from build123d import *

# Parameters (mm, degrees)
SKETCH1_W           = 40
SKETCH1_H           = 70
BOSS_EXTRUDE2_DEPTH = 9
SKETCH3_W           = 20
SKETCH3_H           = 40
CUT_EXTRUDE1_DEPTH  = 42.303752856
SKETCH4_R           = 1.5
CUT_EXTRUDE2_DEPTH  = 42.303752856
SKETCH6_W           = 40
SKETCH6_H           = 5
BOSS_EXTRUDE3_DEPTH = 15
CUT_EXTRUDE3_DEPTH  = 47.914816423
BOSS_EXTRUDE4_DEPTH = 40
SKETCH9_W           = 40
SKETCH9_H           = 5
BOSS_EXTRUDE5_DEPTH = 5
SKETCH10_R          = 1.5
CUT_EXTRUDE4_DEPTH  = 71.887234394
CUT_EXTRUDE5_DEPTH  = 71.887234394
SKETCH12_R          = 1.5
SKETCH12_W          = 20
SKETCH12_H          = 40
BOSS_EXTRUDE6_DEPTH = 3
BOSS_EXTRUDE7_DEPTH = 40
SKETCH14_R          = 1.5
SKETCH14_W          = 20
SKETCH14_H          = 40
BOSS_EXTRUDE8_DEPTH = 2
BOSS_EXTRUDE9_DEPTH = 40
SKETCH17_R          = 2.5
CUT_EXTRUDE6_DEPTH  = 5


with BuildPart() as part:
    # Sketch1 → Boss-Extrude2 (new body)
    with BuildSketch(Plane(origin=(0, 0, 0), x_dir=(0, 0, -1), z_dir=(1, 0, 0))):
        Rectangle(SKETCH1_W, SKETCH1_H)
    extrude(amount=BOSS_EXTRUDE2_DEPTH)

    # Sketch3 → Cut-Extrude1 (cut, through all)
    with BuildSketch(Plane.ZY):
        Rectangle(SKETCH3_W, SKETCH3_H)
    extrude(amount=-CUT_EXTRUDE1_DEPTH, mode=Mode.SUBTRACT)

    # Sketch4 → Cut-Extrude2 (cut, through all)
    with BuildSketch(Plane(origin=(9, 0, 0), x_dir=(0, 0, -1), z_dir=(1, 0, 0))):
        with Locations((-5, -24.5)):
            Circle(SKETCH4_R)
        with Locations((5, -24.5)):
            Circle(SKETCH4_R)
        with Locations((-5, 24.5)):
            Circle(SKETCH4_R)
        with Locations((5, 24.5)):
            Circle(SKETCH4_R)
    extrude(amount=-CUT_EXTRUDE2_DEPTH, mode=Mode.SUBTRACT)

    # Sketch6 → Boss-Extrude3 (add)
    with BuildSketch(Plane.ZY):
        with Locations((0, -32.5)):
            Rectangle(SKETCH6_W, SKETCH6_H)
    extrude(amount=BOSS_EXTRUDE3_DEPTH)

    # Sketch7 → Cut-Extrude3 (cut, through all)
    with BuildSketch(Plane(origin=(9, 0, 0), x_dir=(0, 0, -1), z_dir=(1, 0, 0))):
        with BuildLine():
            Line((-20, 25), (-20, 35))
            Line((-20, 35), (-10, 35))
            ThreePointArc((-10, 35), (-17.071067812, 32.071067812), (-20, 25))
        make_face()
        with BuildLine():
            Line((10, 35), (20, 35))
            Line((20, 35), (20, 25))
            ThreePointArc((20, 25), (17.071067812, 32.071067812), (10, 35))
        make_face()
    extrude(amount=-CUT_EXTRUDE3_DEPTH, mode=Mode.SUBTRACT)

    # Sketch8 → Boss-Extrude4 (add)
    with BuildSketch(Plane(origin=(0, 0, -20), x_dir=(-1, 0, 0), z_dir=(0, 0, -1))):
        Polygon((0, -27), (5, -30), (0, -30), align=None)
    extrude(amount=-BOSS_EXTRUDE4_DEPTH)

    # Sketch9 → Boss-Extrude5 (add)
    with BuildSketch(Plane.ZY.offset(15)):
        with Locations((0, -32.5)):
            Rectangle(SKETCH9_W, SKETCH9_H)
    extrude(amount=BOSS_EXTRUDE5_DEPTH)

    # Sketch10 → Cut-Extrude4 (cut, through all)
    with BuildSketch(Plane(origin=(0, -30, 0), x_dir=(1, 0, 0), z_dir=(0, 1, 0))):
        with Locations(Location((-13, 10, 0), (0, 0, 270))):
            Circle(SKETCH10_R)
        with Locations(Location((-13, -10, 0), (0, 0, 270))):
            Circle(SKETCH10_R)
    extrude(amount=-CUT_EXTRUDE4_DEPTH, mode=Mode.SUBTRACT)

    # Sketch11 → Cut-Extrude5 (cut, through all)
    with BuildSketch(Plane(origin=(0, -30, 0), x_dir=(1, 0, 0), z_dir=(0, 1, 0))):
        with BuildLine():
            add(Edge.make_bspline(
                [(-15, 20), (-17.354348957, 16.495802807), (-19.021015624, 12.650080232), (-20, 8.662193644)],
                knots=[0, 0, 0, 0, 0.292090214, 0.292090214, 0.292090214, 0.292090214], degree=3))
            Line((-15, 20), (-20, 20))
            Line((-20, 20), (-20, 8.662193644))
        make_face()
        with BuildLine():
            add(Edge.make_bspline(
                [(-20, -8.658433055), (-19.021015624, -12.647055954), (-17.354348957, -16.494032059), (-15, -20)],
                knots=[0.707909786, 0.707909786, 0.707909786, 0.707909786, 1, 1, 1, 1], degree=3))
            Line((-20, -8.658433055), (-20, -20))
            Line((-20, -20), (-15, -20))
        make_face()
    extrude(amount=-CUT_EXTRUDE5_DEPTH, mode=Mode.SUBTRACT)

    # Sketch12 → Boss-Extrude6 (add)
    with BuildSketch(Plane.ZY):
        with BuildLine():
            ThreePointArc((-10, 35), (-17.071067812, 32.071067812), (-20, 25))
            Line((-20, 25), (-20, -27))
            Line((-20, -27), (20, -27))
            Line((20, -27), (20, 25))
            ThreePointArc((20, 25), (17.071067812, 32.071067812), (10, 35))
            Line((10, 35), (-10, 35))
        make_face()
        with Locations(Location((-5, 24.5, 0), (0, 0, 180))):
            Circle(SKETCH12_R, mode=Mode.SUBTRACT)
        with Locations(Location((-5, -24.5, 0), (0, 0, 180))):
            Circle(SKETCH12_R, mode=Mode.SUBTRACT)
        with Locations(Location((5, 24.5, 0), (0, 0, 180))):
            Circle(SKETCH12_R, mode=Mode.SUBTRACT)
        with Locations(Location((5, -24.5, 0), (0, 0, 180))):
            Circle(SKETCH12_R, mode=Mode.SUBTRACT)
        Rectangle(SKETCH12_W, SKETCH12_H, mode=Mode.SUBTRACT)
    extrude(amount=BOSS_EXTRUDE6_DEPTH)

    # Sketch13 → Boss-Extrude7 (add)
    with BuildSketch(Plane(origin=(0, 0, -20), x_dir=(-1, 0, 0), z_dir=(0, 0, -1))):
        Polygon((3, -27), (5, -30), (0, -27), align=None)
    extrude(amount=-BOSS_EXTRUDE7_DEPTH)

    # Sketch14 → Boss-Extrude8 (add)
    with BuildSketch(Plane.ZY.offset(3)):
        with BuildLine():
            Line((-20, -27), (20, -27))
            Line((20, -27), (20, 25))
            ThreePointArc((20, 25), (17.071067812, 32.071067812), (10, 35))
            Line((10, 35), (-10, 35))
            ThreePointArc((-10, 35), (-17.071067812, 32.071067812), (-20, 25))
            Line((-20, 25), (-20, -27))
        make_face()
        with Locations(Location((-5, 24.5, 0), (0, 0, 180))):
            Circle(SKETCH14_R, mode=Mode.SUBTRACT)
        with Locations(Location((5, 24.5, 0), (0, 0, 180))):
            Circle(SKETCH14_R, mode=Mode.SUBTRACT)
        with Locations(Location((-5, -24.5, 0), (0, 0, 180))):
            Circle(SKETCH14_R, mode=Mode.SUBTRACT)
        with Locations(Location((5, -24.5, 0), (0, 0, 180))):
            Circle(SKETCH14_R, mode=Mode.SUBTRACT)
        Rectangle(SKETCH14_W, SKETCH14_H, mode=Mode.SUBTRACT)
    extrude(amount=BOSS_EXTRUDE8_DEPTH)

    # Sketch16 → Boss-Extrude9 (add)
    with BuildSketch(Plane(origin=(0, 0, -20), x_dir=(-1, 0, 0), z_dir=(0, 0, -1))):
        Polygon((5, -27), (3, -27), (5, -30), align=None)
    extrude(amount=-BOSS_EXTRUDE9_DEPTH)

    # Sketch17 → Cut-Extrude6 (cut)
    with BuildSketch(Plane(origin=(9, 0, 0), x_dir=(0, 0, -1), z_dir=(1, 0, 0))):
        with Locations((-5, 24.5)):
            Circle(SKETCH17_R)
        with Locations((5, 24.5)):
            Circle(SKETCH17_R)
        with Locations((-5, -24.5)):
            Circle(SKETCH17_R)
        with Locations((5, -24.5)):
            Circle(SKETCH17_R)
    extrude(amount=-CUT_EXTRUDE6_DEPTH, mode=Mode.SUBTRACT)


solid = part.part
Part model, mm, in its own coordinate system. A direction names the side the tool comes from. Round coordinates to 2 decimals unless told otherwise and drop trailing zeros. Write each loop counter-clockwise with the first axis right and the second up, starting at its lowest first coordinate (ties: lowest second). Pieces come first, ordered by that corner, then holes. Notation, with made-up numbers: M 47.25,85.5 L 82.25,85.5 A5 cw 82.25,94.5 Z; hole C 82,16 d9. An arc over 180 degrees is marked long. Return JSON: item names as keys, results as strings. Group by question number.
(1) Saw through at B-B on z = 5. Write the cut outline in (x, y), then the cut area to 3 significant figures.
(2) Saw through at A-A on y = -24.5. Write the cut outline in (x, z).
(3) Saw through at D-D on y = -0.5. Write the cut outline in (x, z).
(4) Two-plate mould, pull along Y, no slides. Class faces 1 (the face through (0, -26, 5)), 2 (the face through (6.54, 26.61, 3.66)), 3 (the face through (3, -5, -20)), 4 (the face through (2.1, 31.99, 17.15)): +Y half, -Y half, draft (parallel to the pull), parting line (faces both ways), or undercut.
(5) Which spindle directions (+Z, -Z, +X, -X, +Y, -Y) get a long thin tool onto all of the face, cutting with end or side? Do faces 5 (the face through (2, -20, 0)), 6 (the face through (6.54, -22.39, 3.66)), 7 (the face through (-5, 2, 13)), 8 (the face through (2, 35, 0)). Say none if no direction does.
(6) Pin check, flat tips, straight feed: pin 1 Ø6.5 at (y, z) = (24.5, -5) entering from -X; pin 2 Ø3.5 at (y, z) = (24.5, 5) entering from +X; pin 3 Ø7.5 at (x, z) = (-15.5, -8) entering from +Y. Stop position of each tip, or through.
(7) Drill centre lines: probe 1 along Y at (x, z) = (-0.75, -5); probe 2 along Z at (x, y) = (1.25, 24.5); probe 3 along Y at (x, z) = (5.2, -5). Where is each one in solid material? Low to high.
(8) Saw through at C-C on x = -13. Write the cut outline in (y, z).
Returned:
{
 "1": {"outline": "M -20,-35 L 9,-35 L 9,-27 L 4,-27 L 4,-26 L -5,-26 L -5,-30 L -20,-30 Z; M -5,-23 L 4,-23 L 4,-22 L 9,-22 L 9,-20 L -5,-20 Z; M -5,20 L 9,20 L 9,22 L 4,22 L 4,23 L -5,23 Z; M -5,26 L 4,26 L 4,27 L 9,27 L 9,35 L -5,35 Z", "area": "391 mm²"},
 "2": {"outline": "M -5,-20 L 9,-20 L 9,-7.5 L 4,-7.5 L 4,-6.5 L -5,-6.5 Z; M -5,-3.5 L 4,-3.5 L 4,-2.5 L 9,-2.5 L 9,2.5 L 4,2.5 L 4,3.5 L -5,3.5 Z; M -5,6.5 L 4,6.5 L 4,7.5 L 9,7.5 L 9,20 L -5,20 Z"},
 "3": {"outline": "M -5,-20 L 9,-20 L 9,-10 L -5,-10 Z; M -5,10 L 9,10 L 9,20 L -5,20 Z"},
 "4": {"face 1": "undercut", "face 2": "undercut", "face 3": "draft", "face 4": "+Y half"},
 "5": {"face 5": "+X, -X", "face 6": "+X", "face 7": "+Z, -Z, -X, +Y", "face 8": "+Z, -Z, +X, -X, +Y"},
 "6": {"pin 1": "x = -5", "pin 2": "x = 4", "pin 3": "y = -30"},
 "7": {"probe 1": "-35 to -26, -23 to -20, 20 to 23, 26 to 35", "probe 2": "-20 to -6.5, -3.5 to 3.5, 6.5 to 20", "probe 3": "-35 to -27, -22 to -20, 20 to 22, 27 to 35"},
 "8": {"outline": "M -35,-20 L -30,-20 L -30,-11.5 L -35,-11.5 Z; M -35,-8.5 L -30,-8.5 L -30,8.5 L -35,8.5 Z; M -35,11.5 L -30,11.5 L -30,20 L -35,20 Z"}
}
